from build123d import *

# Parameters (mm, degrees)
ESBO_O1_W                = 24.6
ESBO_O1_H                = 11
ESBO_O1_W_2              = 20.6
ESBO_O1_H_2              = 7
RESSALTO_EXTRUS_O1_DEPTH = 10
ESBO_O2_R                = 1.8
ESBO_O2_W                = 20.6
ESBO_O2_H                = 7
RESSALTO_EXTRUS_O2_DEPTH = 2
CHANFRO4_SIZE            = 1
CHANFRO2_SIZE            = 1.5
ESBO_O3_W                = 3.653589711
ESBO_O3_H                = 7
ESBO_O3_W_2              = 3.653589584
RESSALTO_EXTRUS_O3_DEPTH = 3
FILETE3_R                = 2


with BuildPart() as part:
    # Esboço1 → Ressalto-extrusão1 (new, symmetric)
    with BuildSketch(Plane.XY):
        Rectangle(ESBO_O1_W, ESBO_O1_H)
        Rectangle(ESBO_O1_W_2, ESBO_O1_H_2, mode=Mode.SUBTRACT)
    extrude(amount=RESSALTO_EXTRUS_O1_DEPTH, both=True)

    # Esboço2 → Ressalto-extrusão2 (add)
    with BuildSketch(Plane(origin=(0, 0, -10), x_dir=(-1, 0, 0), z_dir=(0, 0, -1))):
        Polygon((-12.3, -5.5), (-12.3, 5.5), (-4.5, 12.1), (4.5, 12.1), (12.3, 5.5), (12.3, -5.5), align=None)
        with Locations((-3.05, 8.3)):
            Circle(ESBO_O2_R, mode=Mode.SUBTRACT)
        with Locations(Location((3.05, 8.3, 0), (0, 0, 180))):
            Circle(ESBO_O2_R, mode=Mode.SUBTRACT)
        Rectangle(ESBO_O2_W, ESBO_O2_H, mode=Mode.SUBTRACT)
    extrude(amount=RESSALTO_EXTRUS_O2_DEPTH)

    # Chanfro4
    chanfro4_edges = [part.edges().sort_by_distance(p)[0] for p in [
        (0, 5.5, -10),
    ]]
    chamfer(chanfro4_edges, length=CHANFRO4_SIZE - 0.0001)  # a hair under: the kernel refuses the full size

    # Chanfro2
    chanfro2_edges = [part.edges().sort_by_distance(p)[0] for p in [
        (12.3, 5.5, 0.49995),
        (12.3, -5.5, -1),
        (-12.3, -5.5, -1),
        (-12.3, 5.5, 0.49995),
    ]]
    chamfer(chanfro2_edges, length=CHANFRO2_SIZE)

    # Esboço3 → Ressalto-extrusão3 (add)
    with BuildSketch(Plane.XY.offset(-0.75)):
        with Locations((-5.000000063, 0)):
            Rectangle(ESBO_O3_W, ESBO_O3_H)
        with Locations((5, 0)):
            Rectangle(ESBO_O3_W_2, ESBO_O3_H)
    extrude(amount=-RESSALTO_EXTRUS_O3_DEPTH)

    # Filete3
    filete3_edges = [part.edges().sort_by_distance(p)[0] for p in [
        (-5.000000064, 3.5, -3.75),
        (-5.000000064, -3.5, -3.75),
        (5, 3.5, -3.75),
        (5, -3.5, -3.75),
    ]]
    fillet(filete3_edges, radius=FILETE3_R)


solid = part.part
Build history of the part. All positions in model axes, mm. A direction names the side the tool comes from. Coordinates: 2 decimals unless noted, no trailing zeros. Order: outer loops, then holes, each group sorted by start corner. A loop starts at its lowest first (then second) coordinate and runs counter-clockwise, first axis right, second up. Notation, with made-up numbers: (-20.75, 66) - (36.25, 66) arc R14 ccw to (36.25, 87) - close; hole circle Ø8 at (18.5, -1.75). An arc over 180 degrees is marked (long way). Write item = value, one per line. Start each with the question number.
1) Saw through at B-B on x = 0.5. Write the cut outline in (y, z).
2) Saw through at A-A on z = 3.5. Write the cut outline in (x, y).
3) Two-plate mould, pull along X, no slides. Class faces 1 (the face through (-11.5, -4.8, -0.8)), 2 (the face through (-3.284, 6.515, -10.986)), 3 (the face through (6.827, 0, -2)), 4 (the face through (-0.2, 5.8, -9.3)): pulls with the +X half, pulls with the -X half, needs draft (parallel to the pull), parting line crosses it, or undercut.
4) Flat gauge pins, fed straight in: pin 1 Ø0.9 at (x, y) = (-6, 0.5) entering from -Z; pin 2 Ø1 at (x, z) = (-7, 6.5) entering from +Y; pin 3 Ø1.7 at (x, y) = (2, 8.5) entering from +Z; pin 4 Ø3 at (x, y) = (-3.05, 8.3) entering from +Z. Where does each tip first touch, or does it go through?
5) Wall check: line 1 along Y through (x, z) = (-3.05, -10.9); line 2 along Y through (x, z) = (10.25, -7.75); line 3 along X through (y, z) = (-1.25, -3). Give the ranges that are in metal, low to high. Write a range as from..to.
6) 3-axis set-ups, long thin cutter, end or side, ignore diameter. For faces 5 (the face through (0, 9, -10)), 6 (the face through (11.5, 4.8, 0.6)), 7 (the face through (5, 0, -0.75)), 8 (the face through (3.173, 0, -2)): which of +Z, -Z, +X, -X, +Y, -Y reach the whole face in a straight line?
7) Saw through at D-D on y = -2.5. Write the cut outline in (x, z), then the cut area to 3 significant figures.
8) Saw through at C-C on y = 8.3. Write the cut outline in (x, z), then the cut area to 3 significant figures.
From the geometry:
q1.outline = (-5.5, -12) - (-3.5, -12) - (-3.5, 10) - (-5.5, 10) - close; (3.5, -12) - (12.1, -12) - (12.1, -10) - (6.5, -10) - (5.5, -9) - (5.5, 10) - (3.5, 10) - close
q2.outline = (-12.3, -4) - (-10.8, -5.5) - (10.8, -5.5) - (12.3, -4) - (12.3, 4) - (10.8, 5.5) - (-10.8, 5.5) - (-12.3, 4) - close; hole (-10.3, -3.5) - (10.3, -3.5) - (10.3, 3.5) - (-10.3, 3.5) - close
q3.face_1 = pulls with the -X half
q3.face_2 = undercut
q3.face_3 = undercut
q3.face_4 = needs draft
q4.pin_1 = -3.75
q4.pin_2 = 5.5
q4.pin_3 = -10
q4.pin_4 = through
q5.line_1 = -5.5..-3.5, 3.5..6.5, 10.1..12.1
q5.line_2 = -5.5..-3.5, 3.5..5.5
q5.line_3 = -12.3..-10.3, -6.83..-3.17, 3.17..6.83, 10.3..12.3
q6.face_5 = +Z, +X, -X, +Y
q6.face_6 = +Z, +X, +Y
q6.face_7 = +Z
q6.face_8 = +Z, -Z
q7.outline = (-12.3, -12) - (-10.3, -12) - (-10.3, 10) - (-12.3, 10) - close; (-6.83, -4.02) - (-3.17, -4.02) - (-3.17, -0.75) - (-6.83, -0.75) - close; (3.17, -4.02) - (6.83, -4.02) - (6.83, -0.75) - (3.17, -0.75) - close; (10.3, -12) - (12.3, -12) - (12.3, 10) - (10.3, 10) - close
q7.area = 112 mm^2
q8.outline = (-8.99, -12) - (-4.85, -12) - (-4.85, -10) - (-8.99, -10) - close; (-1.25, -12) - (1.25, -12) - (1.25, -10) - (-1.25, -10) - close; (4.85, -12) - (8.99, -12) - (8.99, -10) - (4.85, -10) - close
q8.area = 21.6 mm^2
